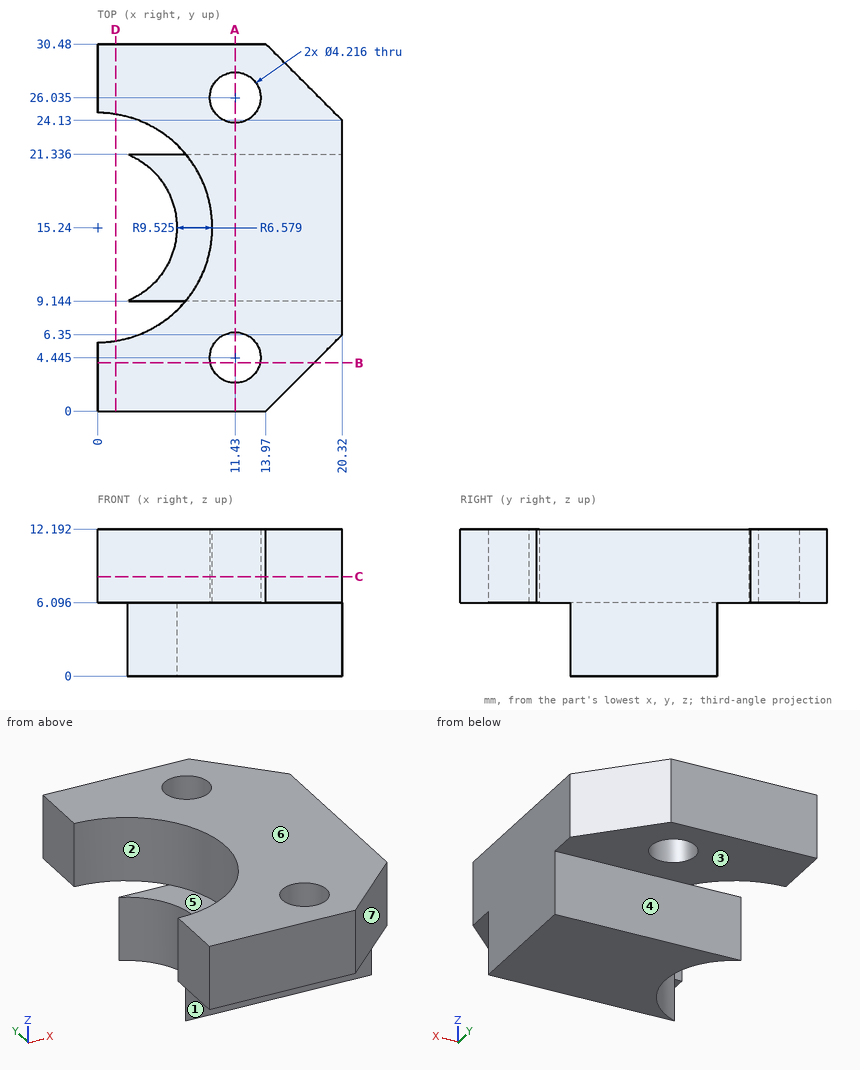
Could you check a few things on this drawing? It's one solid part, dimensions in mm from its lowest x, y, z. A direction names the side the tool comes from. Give positions to 0.01 mm unless a question says otherwise; leave off trailing zeros. Order: outer loops, then holes, each group sorted by start corner. A loop starts at its lowest first (then second) coordinate and runs counter-clockwise, first axis right, second up. Notation, with made-up numbers: (36, 81) - (93, 81) arc R22 ccw to (93, 116) - close; hole circle Ø7 at (34, -5.75). An arc over 180 degrees is marked (long way). One line per question, with ' | ' between items. Start each with the question number.
Item 1: For the marked faces 1, 2 and 3, which set-ups out of +Z, -Z, +X, -X, +Y, -Y let a thin tool reach every point of the face, with its end or its side?
Item 2: I want a section at C-C on z = 8.25. Give the number of separate pieces and of enclosed holes in the cut face.
Item 3: I want a section at B-B on y = 4. Write out the boundary of the cut face in (x, z).
Item 4: I need wall thicknesses on probe 1 along Y at (x, z) = (11.43, 9.25); probe 2 along Y at (x, z) = (9.5, 1.25); probe 3 along Y at (x, z) = (2, 7). Which ranges of each line are inside material? Lowest first, please. Write a range as [from, to].
Item 5: I want a section at A-A on x = 11.43. Write out the boundary of the cut face in (y, z), then the cut area to 3 significant figures.
Item 6: I'm going to push flat-ended pins straight in: pin 1 Ø6.5 at (x, z) = (7, 1.5) entering from -Y; pin 2 Ø8 at (x, y) = (4.5, 18) entering from +Z; pin 3 Ø2.5 at (x, y) = (11.43, 26.035) entering from +Z; pin 4 Ø2 at (x, z) = (10.5, 4) entering from +Y. Where does each tip first touch, or does it pass through?
Item 7: Thinking about a two-plate mould opening in Y: for the marked faces 4, 5, 6 and 7, which applies, pulls with the +Y half, pulls with the -Y half, needs draft (parallel to the pull), parting line crosses it, or undercut?
Item 8: I want a section at D-D on x = 1.5. Write out the boundary of the cut face in (y, z).
Verdict:
1) face 1: -Z, +X, -X, -Y | face 2: +Z, -X | face 3: -Z, +X, -X, +Y
2) separate pieces: 1 | enclosed holes: 2
3) outline: (0, 6.1) - (9.37, 6.1) - (9.37, 12.19) - (0, 12.19) - close; (13.49, 6.1) - (17.97, 6.1) - (17.97, 12.19) - (13.49, 12.19) - close
4) probe 1: [0, 2.34], [6.55, 23.93], [28.14, 30.48] | probe 2: [9.14, 21.34] | probe 3: [0, 5.93], [24.55, 30.48]
5) outline: (0, 6.1) - (2.34, 6.1) - (2.34, 12.19) - (0, 12.19) - close; (6.55, 6.1) - (9.14, 6.1) - (9.14, 0) - (21.34, 0) - (21.34, 6.1) - (23.93, 6.1) - (23.93, 12.19) - (6.55, 12.19) - close; (28.14, 6.1) - (30.48, 6.1) - (30.48, 12.19) - (28.14, 12.19) - close | area: 209 mm^2
6) pin 1: y = 9.14 | pin 2: z = 6.1 | pin 3: through | pin 4: y = 21.34
7) face 4: pulls with the +Y half | face 5: undercut | face 6: needs draft | face 7: pulls with the -Y half
8) outline: (0, 6.1) - (5.83, 6.1) - (5.83, 12.19) - (0, 12.19) - close; (24.65, 6.1) - (30.48, 6.1) - (30.48, 12.19) - (24.65, 12.19) - close
